Geometry: final body of the model. Coordinates: model frame, mm. Round coordinates to 2 decimals unless told otherwise and drop trailing zeros. Write each loop counter-clockwise with the first axis right and the second up, starting at its lowest first coordinate (ties: lowest second). Pieces come first, ordered by that corner, then holes. Notation, with made-up numbers: M 10,36 L 37,36 A35 ccw 37,72 Z; hole C 47.5,35 d6. An arc over 180 degrees is marked long. Use one line per item in the form item = value. Start each with the question number.
Item 1: Pull-direction query (X, two-part tool) for faces 1 (the flat face through (59, 91, 0)), 2 (the flat face through (110, 145, 2)), 3 (the flat face through (73, 145, 2)), 4 (the cylindrical face through (116.99, 2.85, 1.97)); classes: pulls with the +X half, pulls with the -X half, needs draft (parallel to the pull), parting line crosses it, or undercut.
Item 2: Section query C-C (x = 87.5). Return loops of the section in (y, z).
Item 3: Ray query, probe 1 along X at (y, z) = (126, 1.35); probe 2 along X at (y, z) = (101.5, 0.9); probe 3 along Y at (x, z) = (87, 2.15). Return the intervals inside material, ascending.
Item 4: Section query A-A (x = 19). Return loops of the section in (y, z), and give its area (3 significant figures).
Item 5: Section query B-B (y = 122.5). Return loops of the section in (x, z), and give its area (3 significant figures).
Item 6: Section query D-D (x = 47.5). State how many separate pieces and enclosed holes the cut face has, and give its area (3 significant figures).
Item 7: Pin query (flat end, axial travel): pin 1 Ø2 at (y, z) = (34, 2) entering from -X; pin 2 Ø2 at (x, z) = (21, 2) entering from -Y. Return the tip coordinate at first contact, or that it passes through.
from build123d import *

# Parameters (mm, degrees)
SKETCH001_W     = 30
SKETCH001_H     = 4
PAD_DEPTH       = 4
SKETCH002_W     = 20
SKETCH002_H     = 75
SKETCH002_W_2   = 46
SKETCH002_H_2   = 35
POCKET_DEPTH    = 5
SKETCH003_R     = 10.756675
SKETCH003_R_2   = 11.362787
SKETCH003_R_3   = 7.933722
SKETCH003_R_4   = 9.434644
POCKET001_DEPTH = 5


with BuildPart() as part:
    # Sketch001 → Pad (new body)
    with BuildSketch(Plane.XY):
        with BuildLine():
            Line((0, 90), (0, 128.268396))
            ThreePointArc((51.731604, 180), (15.151836, 164.848164), (0, 128.268396))
            Line((51.731604, 180), (110, 180))
            ThreePointArc((120, 170), (117.071068, 177.071068), (110, 180))
            Line((120, 170), (120, 10))
            ThreePointArc((110, 0), (117.071068, 2.928932), (120, 10))
            Line((110, 0), (51.731604, 0))
            ThreePointArc((0, 51.731604), (15.151836, 15.151836), (51.731604, 0))
            Line((0, 51.731604), (0, 90))
        make_face()
        Polygon((100, 60), (100, 38.5), (83, 38.5), (83, 31.5), (100, 31.5), (100, 10), (110, 10), (110, 60), align=None, mode=Mode.SUBTRACT)
        Polygon((100, 120), (110, 120), (110, 170), (100, 170), (100, 148.5), (83, 148.5), (83, 141.5), (100, 141.5), align=None, mode=Mode.SUBTRACT)
        Polygon((73, 37), (43, 37), (43, 33), (73, 33), (73, 35), align=None, mode=Mode.SUBTRACT)
        Polygon((73, 145), (73, 147), (43, 147), (43, 143), (73, 143), align=None, mode=Mode.SUBTRACT)
        with Locations((58, 159)):
            Rectangle(SKETCH001_W, SKETCH001_H, mode=Mode.SUBTRACT)
        with Locations((58, 21)):
            Rectangle(SKETCH001_W, SKETCH001_H, mode=Mode.SUBTRACT)
    extrude(amount=PAD_DEPTH)

    # Sketch002 (on Face45 of Pad) → Pocket (cut)
    with BuildSketch(Plane.XY.offset(4)):
        with Locations((75, 90)):
            Rectangle(SKETCH002_W, SKETCH002_H)
        with Locations((30.894964, 90)):
            Rectangle(SKETCH002_W_2, SKETCH002_H_2)
    extrude(amount=-POCKET_DEPTH, mode=Mode.SUBTRACT)

    # Sketch003 (on Face5 of Pocket) → Pocket001 (cut)
    with BuildSketch(Plane.XY.offset(4)):
        with Locations((46.274479, 126.527054)):
            Circle(SKETCH003_R)
        with Locations((46.274479, 53.472946)):
            Circle(SKETCH003_R)
        with Locations((103.472527, 90)):
            Circle(SKETCH003_R_2)
        with Locations((86.739067, 164.861923)):
            Circle(SKETCH003_R_3)
        with Locations((86.739067, 15.138077)):
            Circle(SKETCH003_R_3)
        with Locations((22.239138, 27.003632)):
            Circle(SKETCH003_R_4)
        with Locations((22.239138, 152.996368)):
            Circle(SKETCH003_R_4)
    extrude(amount=-POCKET001_DEPTH, mode=Mode.SUBTRACT)


solid = part.part
Working result:
q1.face_1 = needs draft
q1.face_2 = undercut
q1.face_3 = undercut
q1.face_4 = pulls with the +X half
q2.outline = M 0,0 L 7.24,0 L 7.24,4 L 0,4 Z; M 23.04,0 L 31.5,0 L 31.5,4 L 23.04,4 Z; M 38.5,0 L 141.5,0 L 141.5,4 L 38.5,4 Z; M 148.5,0 L 156.96,0 L 156.96,4 L 148.5,4 Z; M 172.76,0 L 180,0 L 180,4 L 172.76,4 Z
q3.probe_1 = 0 to 35.53, 57.02 to 65, 85 to 100, 110 to 120
q3.probe_2 = 0 to 7.89, 53.89 to 65, 85 to 120
q3.probe_3 = 0 to 7.21, 23.07 to 31.5, 38.5 to 141.5, 148.5 to 156.93, 172.79 to 180
q4.outline = M 11.67,0 L 18.14,0 L 18.14,4 L 11.67,4 Z; M 35.86,0 L 72.5,0 L 72.5,4 L 35.86,4 Z; M 107.5,0 L 144.14,0 L 144.14,4 L 107.5,4 Z; M 161.86,0 L 168.33,0 L 168.33,4 L 161.86,4 Z
q4.area = 345 mm²
q5.outline = M 0,0 L 36.3,0 L 36.3,4 L 0,4 Z; M 56.25,0 L 65,0 L 65,4 L 56.25,4 Z; M 85,0 L 100,0 L 100,4 L 85,4 Z; M 110,0 L 120,0 L 120,4 L 110,4 Z
q5.area = 280 mm²
q6.separate_pieces = 8
q6.enclosed_holes = 0
q6.area = 344 mm²
q7.pin_1 = 2.78
q7.pin_2 = 9.4
